Print and shaded views of the part. All mm, measured from the part's lowest x, y and z. Coordinates: 2 decimals unless noted, no trailing zeros. Order: outer loops, then holes, each group sorted by start corner. A loop starts at its lowest first (then second) coordinate and runs counter-clockwise, first axis right, second up. Notation, with made-up numbers: (-16, 21.5) -> (9, 21.5) arc R26 ccw to (9, 38.5) -> close; hole circle Ø6 at (71.5, 53.5). An arc over 180 degrees is marked (long way). Write item = value, one per line. Start each with the question number.
Q1. Flat gauge pins, fed straight in: pin 1 (10.5 mm diameter, centred on x = 60, y = 70.5, fed in from +Z); pin 2 (4 mm diameter, centred on x = 50, y = 60.5, fed in from -Z). Where does each tip first touch, or does it go through?
Q2. Wall check: line 1 (X direction, y = 52, z = 3.5); line 2 (X direction, y = 61, z = 4.85). Give the ranges that are in metal, low to high. Write a range as from..to.
Q3. Cut at A-A, the plane y = 70.5. List the corners of the cut face in (x, z).
Q4. Cut at B-B, the plane x = 50. Give the number of separate pieces and of enclosed holes in the cut face, plus the area to 3 significant figures.
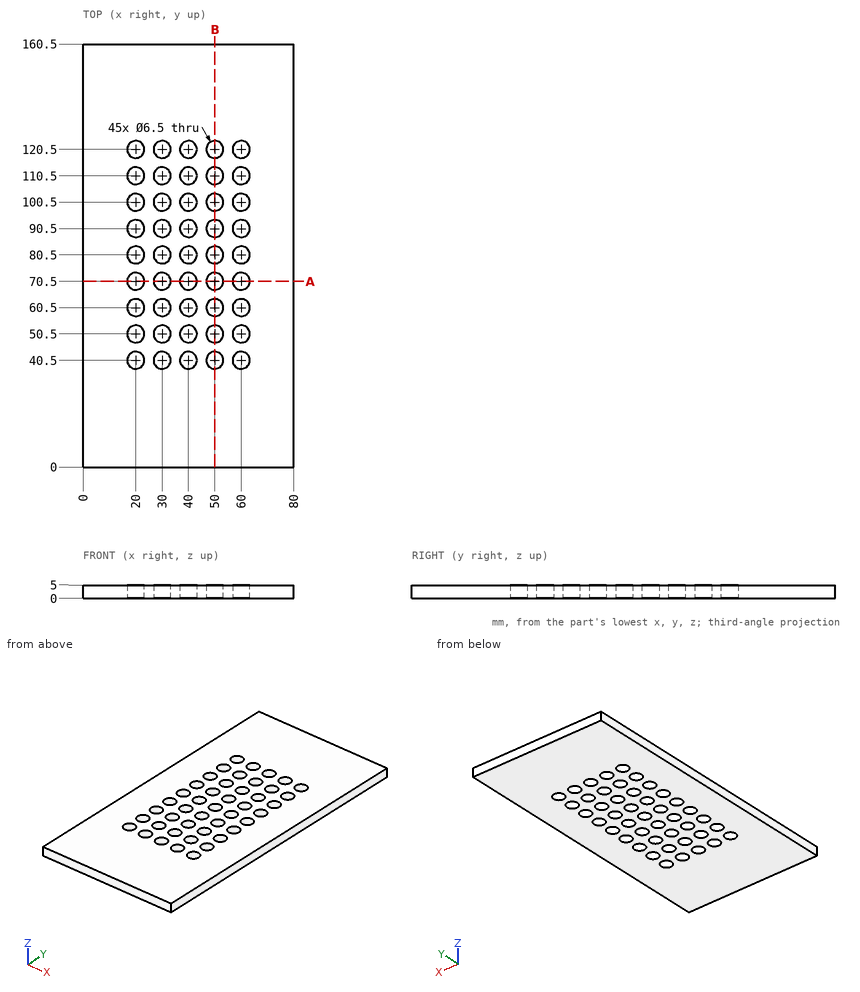
Here are the results:
q1.pin_1 = 5
q1.pin_2 = through
q2.line_1 = 0..17.12, 22.88..27.12, 32.88..37.12, 42.88..47.12, 52.88..57.12, 62.88..80
q2.line_2 = 0..16.79, 23.21..26.79, 33.21..36.79, 43.21..46.79, 53.21..56.79, 63.21..80
q3.outline = (0, 0) -> (16.75, 0) -> (16.75, 5) -> (0, 5) -> close; (23.25, 0) -> (26.75, 0) -> (26.75, 5) -> (23.25, 5) -> close; (33.25, 0) -> (36.75, 0) -> (36.75, 5) -> (33.25, 5) -> close; (43.25, 0) -> (46.75, 0) -> (46.75, 5) -> (43.25, 5) -> close; (53.25, 0) -> (56.75, 0) -> (56.75, 5) -> (53.25, 5) -> close; (63.25, 0) -> (80, 0) -> (80, 5) -> (63.25, 5) -> close
q4.separate_pieces = 10
q4.enclosed_holes = 0
q4.area = 510 mm²
